```python
from build123d import *

# Parameters (mm, degrees)
SKETCH1_R           = 4
BOSS_EXTRUDE1_DEPTH = 30
CUT_EXTRUDE3_START  = -15
CUT_EXTRUDE3_DEPTH  = 15


with BuildPart() as part:
    # Sketch1 → Boss-Extrude1 (new body)
    with BuildSketch(Plane.XY):
        with BuildLine():
            Line((0, -10), (60, -10))
            Line((60, -10), (60, 50))
            ThreePointArc((60, 50), (50, 60), (40, 50))
            Line((40, 50), (0, 10))
            ThreePointArc((0, 10), (-10, 0), (0, -10))
        make_face()
        with Locations((50, 50)):
            Circle(SKETCH1_R, mode=Mode.SUBTRACT)
        Circle(SKETCH1_R, mode=Mode.SUBTRACT)
    extrude(amount=BOSS_EXTRUDE1_DEPTH)

    # Sketch3 → Cut-Extrude3 (cut)
    with BuildSketch(Plane.XY.offset(30).offset(CUT_EXTRUDE3_START)):
        with BuildLine():
            Line((60, -217.989898732), (60, -10))
            Line((60, -10), (60, 50))
            ThreePointArc((60, 50), (50, 60), (40, 50))
            Line((40, 50), (0, 10))
            ThreePointArc((0, 10), (-10, 0), (0, -10))
            Line((0, -10), (60, -10))
            Line((60, -10), (25, -10))
            Line((25, -10), (25, 35))
            Line((25, 35), (25, 242.989898732))
            Line((25, 242.989898732), (-389.785969286, 211.497176047))
            Line((-389.785969286, 211.497176047), (-354.785969286, -249.482621417))
            Line((-354.785969286, -249.482621417), (60, -217.989898732))
        make_face()
    extrude(amount=CUT_EXTRUDE3_DEPTH, mode=Mode.SUBTRACT)


solid = part.part
```
Design review of the part built by this model. Coordinates are the model's own, in mm. A direction names the side the tool comes from. Round coordinates to 2 decimals unless told otherwise and drop trailing zeros. Write each loop counter-clockwise with the first axis right and the second up, starting at its lowest first coordinate (ties: lowest second). Pieces come first, ordered by that corner, then holes.
Item 1: For faces 4 (the flat face through (25, 12, 22)), 5 (the cylindrical face through (-0.867, -3.905, 7.395)), list the 3-axis set-ups (+Z, -Z, +X, -X, +Y, -Y) from which the entire face can be reached by the end or side of a thin tool; tool diameter is ignored.
Item 2: We need section D-D on z = 22.5. Write out the cut boundary in (x, y), and give its area (3 significant figures).
Item 3: We need section B-B on x = 50. Write out the cut boundary in (y, z), and give its area (3 significant figures).
Item 4: For probe 1 along Y at (x, z) = (0, 11.25); probe 2 along X at (y, z) = (0, 4); probe 3 along X at (y, z) = (22.5, 23), list the stretches that pass through material, from the lowest coordinate up.
Item 5: Clearance check with flat-ended pins moving along their axes: pin 1 Ø4.5 at (y, z) = (3, 24.5) entering from -X; pin 2 Ø8 at (x, y) = (18, 39) entering from -Z; pin 3 Ø8 at (x, z) = (-1.5, 11.5) entering from +Y; pin 4 Ø12 at (y, z) = (37.5, 20) entering from -X. State where each tip first meets the part, or that it passes through.
Item 6: We need section C-C on z = 8.25. Write out the cut boundary in (x, y), and give its area (3 significant figures).
Item 7: The part is to be moulded in two halves that separate along Y. For faces 1 (the flat face through (42, 18, 30)), 2 (the cylindrical face through (46.8, 47.6, 14.8)), 3 (the cylindrical face through (50, 60, 15)), say which applies: +Y half, -Y half, draft (parallel to the pull), parting line (faces both ways), or undercut.
Item 8: We need section A-A on y = 0. Write out the cut boundary in (x, z).
Returned:
1. face 4: +Z, -X, +Y, -Y
1. face 5: +Z, -Z
2. outline: (25, -10) - (60, -10) - (60, 50) arc R10 ccw to (40, 50) - (25, 35) - close; hole circle Ø8 at (50, 50)
2. area: 2,090 mm2
3. outline: (-10, 0) - (46, 0) - (46, 30) - (-10, 30) - close; (54, 0) - (60, 0) - (60, 30) - (54, 30) - close
3. area: 1,860 mm2
4. probe 1: y = -10 to -4, 4 to 10
4. probe 2: x = -10 to -4, 4 to 60
4. probe 3: x = 25 to 60
5. pin 1: stops at x = 25
5. pin 2: passes through
5. pin 3: stops at y = 12.5
5. pin 4: stops at x = 24.18
6. outline: (0, -10) - (60, -10) - (60, 50) arc R10 ccw to (40, 50) - (0, 10) arc R10 ccw to start; hole circle Ø8 at (0, 0); hole circle Ø8 at (50, 50)
6. area: 3,010 mm2
7. face 1: draft
7. face 2: undercut
7. face 3: +Y half
8. outline: (-10, 0) - (-4, 0) - (-4, 15) - (-10, 15) - close; (4, 0) - (60, 0) - (60, 30) - (25, 30) - (25, 15) - (4, 15) - close
